Answer from the drawing. Dimensions are ordinates in mm from the lowest x, y and z of the part. Round coordinates to 2 decimals unless told otherwise and drop trailing zeros. Loops run counter-clockwise (first coordinate to the right, second up) from the corner with the lowest first, then second, coordinate; pieces in that order, holes last. Notation, with made-up numbers: M 31,1 L 62,1 A8 cw 62,15 Z; hole C 47,-32 d3. An arc over 180 degrees is marked long. Answer as a JSON object with one key per item and string values.
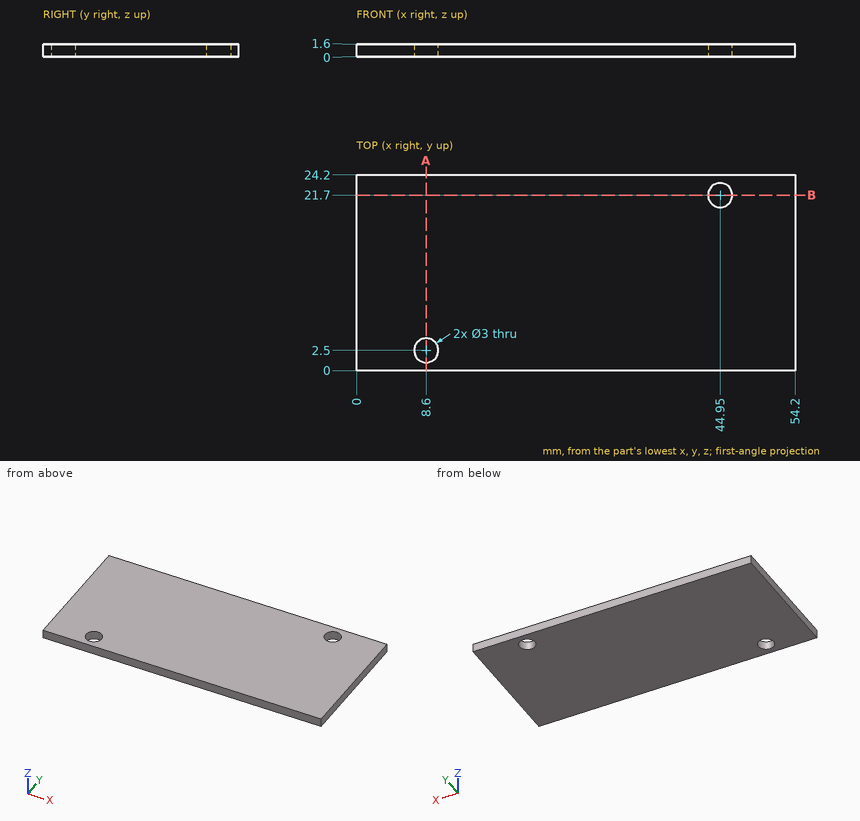
Item 1: The part is cut by section B-B (y = 21.7). Give the vertices of the cut face in (x, z), then the cut area to 3 significant figures.
Values follow:
{"outline": "M 0,0 L 43.45,0 L 43.45,1.6 L 0,1.6 Z; M 46.45,0 L 54.2,0 L 54.2,1.6 L 46.45,1.6 Z", "area": "81.9 mm^2"}
Item 2: Straight lines are drawn through the part: line 1 (Y direction, x = 8.6, z = 1.2); line 2 (X direction, y = 21, z = 0.7); line 3 (Y direction, x = 7.5, z = 0.5). For each, find the intervals that lie inside material, in ascending order.
Values follow:
{"line 1": "0 to 1, 4 to 24.2", "line 2": "0 to 43.62, 46.28 to 54.2", "line 3": "0 to 1.48, 3.52 to 24.2"}
Item 3: The part is cut by section A-A (x = 8.6). Give the vertices of the cut face in (y, z), then the cut area to 3 significant figures.
Values follow:
{"outline": "M 0,0 L 1,0 L 1,1.6 L 0,1.6 Z; M 4,0 L 24.2,0 L 24.2,1.6 L 4,1.6 Z", "area": "33.9 mm^2"}
Item 4: A flat-ended cylindrical pin translates along its axis: P1, Ø1, axis at x = 33, y = 20.5, coming from the -Z side. Find the tip coordinate at first contact, or state that the pin passes through.
Values follow:
{"P1": "z = 0"}
